Could you check a few things on this drawing? It's one solid part, dimensions in mm from its lowest x, y, z. A direction names the side the tool comes from. Coordinates: 2 decimals unless noted, no trailing zeros. Write each loop counter-clockwise with the first axis right and the second up, starting at its lowest first coordinate (ties: lowest second). Pieces come first, ordered by that corner, then holes.
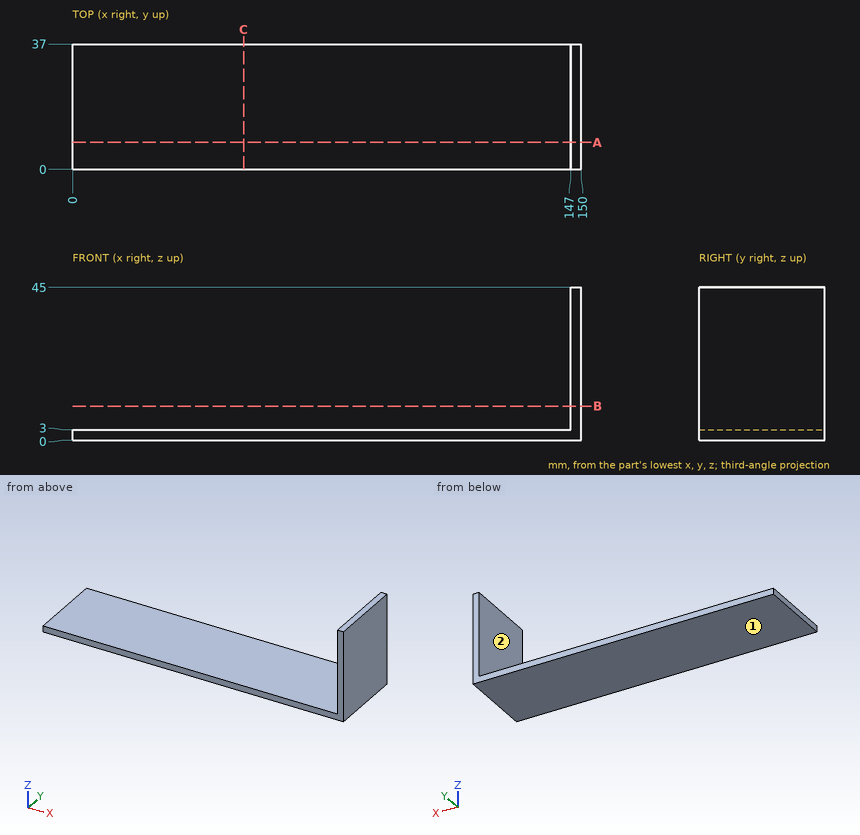
1) Imagine slicing it at A-A on y = 8. Please give me the cut outline in (x, z), then the cut area to 3 significant figures.
Values follow:
outline: (0, 0) - (150, 0) - (150, 45) - (147, 45) - (147, 3) - (0, 3) - close
area: 576 mm2
2) On a 3-axis mill with a long thin cutter (end or side, diameter ignored), from which of +Z, -Z, +X, -X, +Y, -Y can I reach the whole of each face in a straight line? I mean the marked faces 1 and 2. Say none if no direction works.
Values follow:
face 1: -Z, +X, -X, +Y, -Y
face 2: +Z, -X, +Y, -Y
3) Will these pins go through, and if not, where does the flat tip stop? pin 1 (4 mm diameter, centred on x = 79, y = 14.5, fed in from +Z); pin 2 (18.5 mm diameter, centred on y = 27, z = 20.5, fed in from -X).
Values follow:
pin 1: stops at z = 3
pin 2: stops at x = 147
4) Imagine slicing it at C-C on x = 50.5. Please give me the cut outline in (y, z), then the cut area to 3 significant figures.
Values follow:
outline: (0, 0) - (37, 0) - (37, 3) - (0, 3) - close
area: 111 mm2
5) Imagine slicing it at B-B on z = 10. Please give me the cut outline in (x, y).
Values follow:
outline: (147, 0) - (150, 0) - (150, 37) - (147, 37) - close
6) I need wall thicknesses on probe 1 along Z at (x, y) = (127.5, 10); probe 2 along X at (y, z) = (9, 17.5). Which ranges of each line are inside material? Lowest first, please.
Values follow:
probe 1: z = 0 to 3
probe 2: x = 147 to 150
